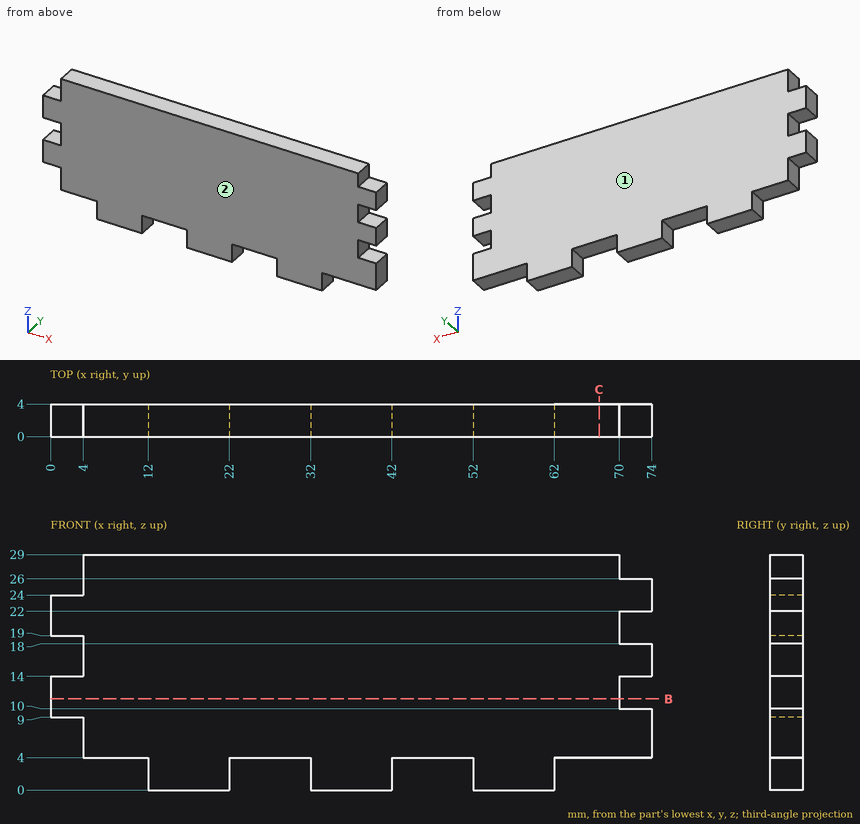
Drawing for the job (mm, zero at the part's lowest x, y, z). Coordinates: 2 decimals unless noted, no trailing zeros. Order: outer loops, then holes, each group sorted by start corner. A loop starts at its lowest first (then second) coordinate and runs counter-clockwise, first axis right, second up. Notation, with made-up numbers: (-14.5, -37.5) - (-10.5, -37.5) arc R11 cw to (-10.5, -26.5) - close; hole circle Ø5 at (-24.5, 13). An arc over 180 degrees is marked (long way). Use a Markdown table: item, result. Add a question column.
(1) Flat gauge pins, fed straight in: pin 1 (2 mm diameter, centred on x = 71, y = 1.5, fed in from -Z); pin 2 (2 mm diameter, centred on x = 72.5, y = 2.5, fed in from +Z); pin 3 (1.2 mm diameter, centred on y = 3, z = 6, fed in from -X). Where does each tip first touch, or does it go through?
(2) Pull direction Y, two halves, no side cores. Call the marked faces 1 and 2: +Y half, -Y half, draft (parallel to the pull), parting line (faces both ways), or undercut.
(3) Saw through at C-C (x = 67.5). Give the cut face in (y, z), then the cut area to 3 significant figures.
(4) Drill centre lines: line 1 along X through (y, z) = (2.55, 24.75); line 2 along Z through (x, y) = (31, 1.4); line 3 along X through (y, z) = (3.7, 20.75). Where is each one in solid material? Low to high. Write a range as [from, to].
(5) Saw through at B-B (z = 11.25). Give the cut face in (x, y).
Solved:
| question | item | result |
|---|---|---|
| 1 | pin 1 | stops at z = 4 |
| 1 | pin 2 | stops at z = 26 |
| 1 | pin 3 | stops at x = 4 |
| 2 | face 1 | +Y half |
| 2 | face 2 | -Y half |
| 3 | outline | (0, 4) - (4, 4) - (4, 29) - (0, 29) - close |
| 3 | area | 100 mm² |
| 4 | line 1 | x = [4, 74] |
| 4 | line 2 | z = [4, 29] |
| 4 | line 3 | x = [0, 70] |
| 5 | outline | (0, 0) - (70, 0) - (70, 4) - (0, 4) - close |
